For this review, take the finished solid that the model builds, in its own axes (mm). Round coordinates to 2 decimals unless told otherwise and drop trailing zeros. Write each loop counter-clockwise with the first axis right and the second up, starting at its lowest first coordinate (ties: lowest second). Pieces come first, ordered by that corner, then holes.
from build123d import *

# Parameters (mm, degrees)
SKETCH_W  = 10
SKETCH_H  = 10
PAD_DEPTH = 5


with BuildPart() as part:
    # Sketch → Pad (new body, symmetric)
    with BuildSketch(Plane.XZ):
        with Locations((0, 5)):
            Rectangle(SKETCH_W, SKETCH_H)
    extrude(amount=PAD_DEPTH, both=True)

    # Sketch001 → Revolution (revolve)
    with BuildSketch(Plane.XZ):
        with BuildLine():
            ThreePointArc((0, 9.64162), (4.75, 14.39162), (0, 19.14162))
            Line((0, 19.14162), (0, 9.64162))
        make_face()
    revolve(axis=Axis((0, 0, 0), (0, 0, 1)))


solid = part.part
(1) We need section B-B, the plane y = -3.5. Give the boundary of the cut face in (x, z).
Geometry check:
outline: (-5, 0) - (5, 0) - (5, 10) - (-5, 10) - close; circle Ø6.42 at (0, 14.39)
(2) Mouldability with a two-part tool opening along Z and no side actions: class faces 1 (the face through (0, 0, 0)), 2 (the face through (0, 5, 5)), 3 (the face through (2.2, -0.1, 10)) as pulls with the +Z half, pulls with the -Z half, needs draft (parallel to the pull), parting line crosses it, or undercut.
Geometry check:
face 1: pulls with the -Z half
face 2: needs draft
face 3: undercut
(3) We need section C-C, the plane x = -0.5. Give the boundary of the cut face in (y, z), and give its area (3 significant figures).
Geometry check:
outline: (-5, 0) - (5, 0) - (5, 10) - (1.74, 10) arc R4.72 ccw (long way) to (-1.74, 10) - (-5, 10) - close
area: 169 mm2
(4) We need section A-A, the plane x = -3.25. Give the boundary of the cut face in (y, z).
Geometry check:
outline: (-5, 0) - (5, 0) - (5, 10) - (-5, 10) - close; circle Ø6.93 at (0, 14.39)
(5) For pin 1 Ø3 at (x, z) = (3, 14) entering from -Y; pin 2 Ø5 at (x, y) = (3, -3) entering from +Z; pin 3 Ø5 at (y, z) = (1.5, 14) entering from -X, all flat-tipped, find the tip position at first contact; note any pin that passes through.
Geometry check:
pin 1: stops at y = -4.5
pin 2: stops at z = 18.81
pin 3: stops at x = -4.75
(6) For line 1 along Z through (x, y) = (0, 3.75); line 2 along Z through (x, y) = (-2, 2.75) (3 decimals); line 3 along Z through (x, y) = (-3.5, -4.25), list the stretches that pass through material, from the lowest coordinate up.
Geometry check:
line 1: z = 0 to 10, 11.48 to 17.31
line 2: z = 0 to 10, 11.075 to 17.708
line 3: z = 0 to 10
